Check sheet for the modelled part. Datum: model origin and axes. Units: mm. A direction names the side the tool comes from. Round coordinates to 2 decimals unless told otherwise and drop trailing zeros. Loops run counter-clockwise (first coordinate to the right, second up) from the corner with the lowest first, then second, coordinate; pieces in that order, holes last. Notation, with made-up numbers: (80, 56) - (105, 56) arc R10 ccw to (105, 75) - close; hole circle Ø6 at (-36.75, -30.75). An arc over 180 degrees is marked (long way). Put each result on its own line as item: value. Start each with the question number.
Item 1: Section check A-A, the plane x = 19.5. Record the cut outline in (y, z).
Item 2: Section check C-C, the plane z = -1. Record the cut outline in (x, y), and give its area (3 significant figures).
Item 3: Tool access check on faces 1 (the flat face through (-29.25, -1, -22)), 2 (the flat face through (0, 11, -28)), 3 (the flat face through (3.45, -1, 22)), 4 (the flat face through (-15, -1, -24)). Record the directions out of +Z, -Z, +X, -X, +Y, -Y that give a thin tool (end or side, any length) a straight path to the whole face; none if there is none.
Item 4: Gauge pin test, flat ends, axial feed: pin 1 Ø1.5 at (y, z) = (-1.5, -22) entering from -X; pin 2 Ø2.5 at (y, z) = (-1, -20.5) entering from +X; pin 3 Ø1.5 at (y, z) = (-2, 22) entering from +X; pin 4 Ø2.5 at (x, y) = (-19, -1.5) entering from -Z. Record the tip position at first contact, or that the pin passes through.
Item 5: Section check B-B, the plane y = 7.25. Record the cut outline in (x, z), and give its area (3 significant figures).
Item 6: Draft check along X on faces 5 (the flat face through (0, 11, 28)), 6 (the flat face through (-13, -1, 24)), 7 (the flat face through (35.75, 10, 0)). Enter one of: pulls with the +X half, pulls with the -X half, needs draft (parallel to the pull), parting line crosses it, or undercut.
Item 7: Material ranges on line 1 along Z through (x, y) = (-9, 9.5); line 2 along X through (y, z) = (17.5, 1.5); line 3 along Y through (x, z) = (-10.5, -14.5), recorded low to high.
Item 8: Section check D-D, the plane x = -22. Record the cut outline in (y, z), and give its area (3 significant figures).
from build123d import *

# Parameters (mm, degrees)
CROQUIS1_W              = 71.5
CROQUIS1_H              = 60
SALIENTE_EXTRUIR1_DEPTH = 20
VACIADO1_T              = -2
CROQUIS3_W              = 32.700305435
CROQUIS3_H              = 4.402483211
CROQUIS3_W_2            = 29.112946205
CROQUIS3_H_2            = 4.942332104
SALIENTE_EXTRUIR2_DEPTH = 3


with BuildPart() as part:
    # Croquis1 → Saliente-Extruir1 (new body)
    with BuildSketch(Plane(origin=(0, 0, 0), x_dir=(1, 0, 0), z_dir=(0, 1, 0))):
        Rectangle(CROQUIS1_W, CROQUIS1_H)
    extrude(amount=SALIENTE_EXTRUIR1_DEPTH)

    # Vaciado1
    vaciado1_openings = [part.faces().sort_by_distance(p)[0] for p in [
        (0, 20, 0),
    ]]
    offset(amount=VACIADO1_T, openings=vaciado1_openings, kind=Kind.INTERSECTION)

    # Croquis3 → Saliente-Extruir2 (add)
    with BuildSketch(Plane.XZ):
        with Locations((-12.899847283, 21.798758394)):
            Rectangle(CROQUIS3_W, CROQUIS3_H)
        with Locations((-14.693526898, -21.528833948)):
            Rectangle(CROQUIS3_W_2, CROQUIS3_H_2)
    extrude(amount=SALIENTE_EXTRUIR2_DEPTH)


solid = part.part
Check result:
1. outline: (0, -30) - (20, -30) - (20, -28) - (2, -28) - (2, 28) - (20, 28) - (20, 30) - (0, 30) - close
2. outline: (-35.75, 0) - (35.75, 0) - (35.75, 20) - (33.75, 20) - (33.75, 2) - (-33.75, 2) - (-33.75, 20) - (-35.75, 20) - close
2. area: 215 mm²
3. face 1: +Z, -Z, -X, -Y
3. face 2: +Y
3. face 3: +Z, -Z, +X, -Y
3. face 4: -Z, +X, -X, -Y
4. pin 1: x = -29.25
4. pin 2: x = 35.75
4. pin 3: x = 3.45
4. pin 4: z = -24
5. outline: (-35.75, -30) - (35.75, -30) - (35.75, 30) - (-35.75, 30) - close; hole (-33.75, -28) - (33.75, -28) - (33.75, 28) - (-33.75, 28) - close
5. area: 510 mm²
6. face 5: undercut
6. face 6: needs draft
6. face 7: pulls with the +X half
7. line 1: -30 to -28, 28 to 30
7. line 2: -35.75 to -33.75, 33.75 to 35.75
7. line 3: 0 to 2
8. outline: (-3, -24) - (0, -24) - (0, -30) - (20, -30) - (20, -28) - (2, -28) - (2, 28) - (20, 28) - (20, 30) - (0, 30) - (0, 24) - (-3, 24) - (-3, 19.6) - (0, 19.6) - (0, -19.06) - (-3, -19.06) - close
8. area: 220 mm²
